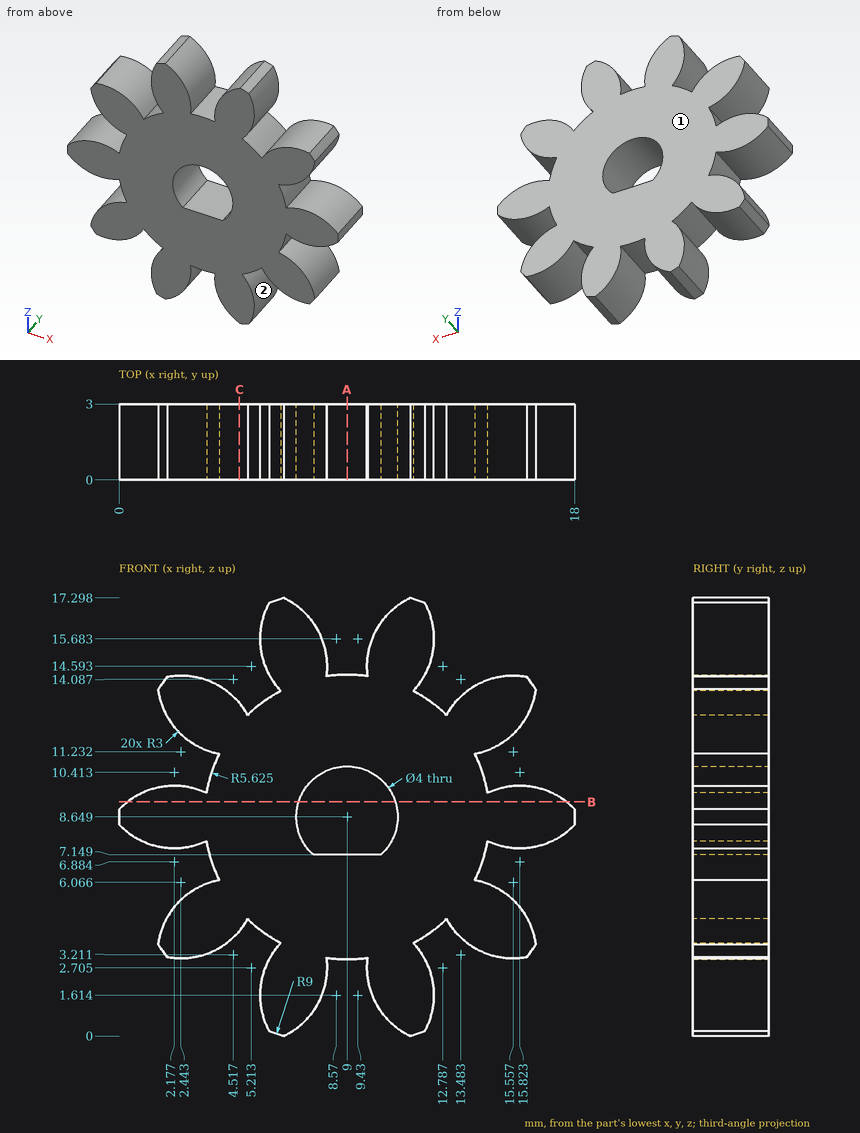
Drawing for the job (mm, zero at the part's lowest x, y, z). Coordinates: 2 decimals unless noted, no trailing zeros. Order: outer loops, then holes, each group sorted by start corner. A loop starts at its lowest first (then second) coordinate and runs counter-clockwise, first axis right, second up.
Item 1: Drill centre lines: L1, parallel to Z at x = 10.5, y = 2.15 (1 decimal); L2, parallel to X at y = 0.2, z = 1.75; L3, parallel to X at y = 1, z = 8.25. Where is each one in solid material? Low to high.
Check sheet entries:
L1: z = 0.8 to 7.3, 10 to 16.5
L2: x = 5.57 to 8.06, 9.94 to 12.43
L3: x = 0.1 to 7.04, 10.96 to 17.9
Item 2: Band-saw the part on A-A on x = 9. List the corners of the cut face in (y, z).
Check sheet entries:
outline: (0, 3.02) - (3, 3.02) - (3, 7.15) - (0, 7.15) - close; (0, 10.65) - (3, 10.65) - (3, 14.27) - (0, 14.27) - close
Item 3: Pin check, flat tip, straight feed: pin 1 Ø1.5 at (y, z) = (1.5, 13) entering from +X. Stop position of the tip, or through.
Check sheet entries:
pin 1: stops at x = 16.46
Item 4: Two-plate mould, pull along Z, no slides. Class the marked faces 1 and 2: +Z half, -Z half, draft (parallel to the pull), parting line (faces both ways), or undercut.
Check sheet entries:
face 1: draft
face 2: undercut
Item 5: Band-saw the part on C-C on x = 4.75. List the corners of the cut face in (y, z), plus the area to 3 significant figures.
Check sheet entries:
outline: (0, 4.15) - (3, 4.15) - (3, 13.15) - (0, 13.15) - close
area: 27.0 mm2
Item 6: Band-saw the part on B-B on z = 9.25. List the corners of the cut face in (x, y).
Check sheet entries:
outline: (0.33, 0) - (7.09, 0) - (7.09, 3) - (0.33, 3) - close; (10.91, 0) - (17.67, 0) - (17.67, 3) - (10.91, 3) - close
